from build123d import *

# Parameters (mm, degrees)
F0_W     = 1879.6
F0_H     = 762
F1_DEPTH = 127
F2_W     = 1778
F2_H     = 711.2
F3_DEPTH = 635
F4_R     = 25.4
F5_DEPTH = 762.001


# Not quite as in the source:
# - a feature names something its author has since deleted; it is built from what else it names


with BuildPart() as f1:
    # F0 (on Top) → F1 (new body, symmetric)
    with BuildSketch(Plane.XY):
        Rectangle(F0_W, F0_H)
    extrude(amount=F1_DEPTH, both=True)

    # F2 (on face) → F3 (cut, symmetric)
    with BuildSketch(Plane.XY.offset(127)):
        Rectangle(F2_W, F2_H)
    extrude(amount=F3_DEPTH, both=True, mode=Mode.SUBTRACT)

    # F4 (on face) → F5 (cut, through all)
    with BuildSketch(Plane.XZ.offset(381)):
        with Locations((-762, 0)):
            Circle(F4_R)
        with Locations((762, 0)):
            Circle(F4_R)
        Circle(F4_R)
    extrude(amount=-F5_DEPTH, mode=Mode.SUBTRACT)


solid = f1.part
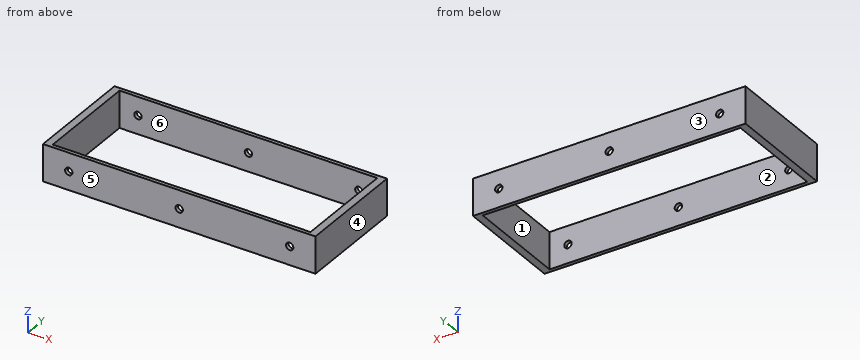
Could you check a few things on this model? Use its own coordinates, in mm. Face numbers are marked on the shaded views. A direction names the side the tool comes from. Round coordinates to 2 decimals unless told otherwise and drop trailing zeros. Order: outer loops, then holes, each group sorted by start corner. A loop starts at its lowest first (then second) coordinate and runs counter-clockwise, first axis right, second up.
(1) Imagine slicing it at B-B (x = -614.5). Write out the boundary of the cut face in (y, z).
Response values:
outline: (-381, -127) - (-355.6, -127) - (-355.6, 127) - (-381, 127) - close; (355.6, -127) - (381, -127) - (381, 127) - (355.6, 127) - close
(2) Which directions (+Z, -Z, +X, -X, +Y, -Y) give clear straight access to the entire face, cutting with the end or side of a thin tool? Please do the marked faces 5 and 6.
Response values:
face 5: +Z, -Z, +X, -X, -Y
face 6: +Z, -Z
(3) Imagine slicing it at A-A (z = 0). Count the separate pieces of the cut face and the enclosed holes in it, plus the area to 3 significant figures.
Response values:
separate pieces: 6
enclosed holes: 0
area: 160,000 mm2
(4) If we mould it in two halves opening along Y, with no side actions, what happens to the marked faces 1, 2, 3 and 4? For each: released by +Y, released by -Y, zero draft, split by the parting line, or undercut.
Response values:
face 1: undercut
face 2: undercut
face 3: released by +Y
face 4: zero draft
(5) Please list where these lines run through material, in increasing order: line 1 along Z through (x, y) = (762, 367.75); line 2 along Y through (x, z) = (-368.5, 46); line 3 along X through (y, z) = (-13, -12.5).
Response values:
line 1: z = -127 to -25.4, 25.4 to 127
line 2: y = -381 to -355.6, 355.6 to 381
line 3: x = -939.8 to -889, 889 to 939.8
(6) Imagine slicing it at C-C (y = -24.5). Write out the boundary of the cut face in (x, z).
Response values:
outline: (-939.8, -127) - (-889, -127) - (-889, 127) - (-939.8, 127) - close; (889, -127) - (939.8, -127) - (939.8, 127) - (889, 127) - close
